Answer from the drawing. Dimensions are ordinates in mm from the lowest x, y and z of the part. Give positions to 0.01 mm unless a question says otherwise; leave off trailing zeros. Loops run counter-clockwise (first coordinate to the right, second up) from the corner with the lowest first, then second, coordinate; pieces in that order, holes last. Notation, with made-up numbers: (-7, -28) -> (39, -28) arc R15 cw to (39, -10) -> close; hole circle Ø8 at (83, 42.25). An arc over 180 degrees is marked (long way). Write each question's results on one line, items separated by ' | '. Start each with the question number.
Item 1: Section A-A on y = 41.5 is taken. Write down the section's boundary in (x, z).
Item 2: Section C-C on z = 25.5 is taken. Write down the section's boundary in (x, y), and give its area (3 significant figures).
Item 3: Section B-B on x = 3.75 is taken. Write down the section's boundary in (y, z).
Item 4: Each of these flat-tipped pins is pushed along its axis until it touches: P1, Ø2.5, axis at x = 3.5, y = 98.5, coming from the +Z side; P2, Ø2.5, axis at x = 3.5, z = 7.5, coming from the +Y side; P3, Ø1.6, axis at x = 4, y = 98.5, coming from the -Z side. Where does it stop, or does it pass through?
Item 5: Find the intervals of material crossed by line 1 (Z direction, x = 0.35, y = 34.5); line 2 (Z direction, x = 0.9, y = 97); line 3 (Y direction, x = 2.15, z = 41), in increasing order.
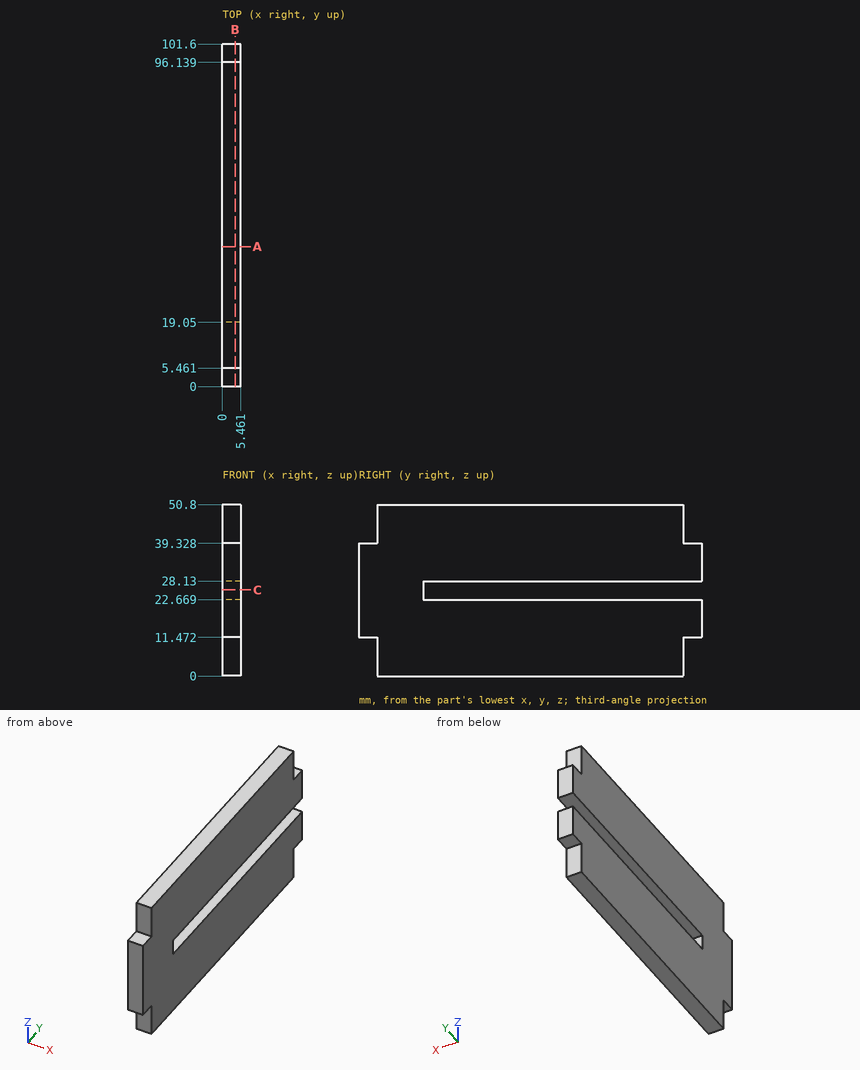
Findings:
1) outline: (0, 0) -> (5.46, 0) -> (5.46, 22.67) -> (0, 22.67) -> close; (0, 28.13) -> (5.46, 28.13) -> (5.46, 50.8) -> (0, 50.8) -> close
2) outline: (0, 0) -> (5.46, 0) -> (5.46, 19.05) -> (0, 19.05) -> close | area: 104 mm2
3) outline: (0, 11.47) -> (5.46, 11.47) -> (5.46, 0) -> (96.14, 0) -> (96.14, 11.47) -> (101.6, 11.47) -> (101.6, 22.67) -> (19.05, 22.67) -> (19.05, 28.13) -> (101.6, 28.13) -> (101.6, 39.33) -> (96.14, 39.33) -> (96.14, 50.8) -> (5.46, 50.8) -> (5.46, 39.33) -> (0, 39.33) -> close
4) P1: z = 39.33 | P2: y = 96.14 | P3: z = 11.47
5) line 1: 0 to 22.67, 28.13 to 50.8 | line 2: 11.47 to 22.67, 28.13 to 39.33 | line 3: 5.46 to 96.14
